Input: part model. Units: mm. Frame: model coordinates. A direction names the side the tool comes from. Coordinates: 2 decimals unless noted, no trailing zeros. Use one line per item in the form item = value.
from build123d import *

# Parameters (mm, degrees)
SKETCH_R              = 40
PAD_DEPTH             = 8
SKETCH001_R           = 1.5
POCKET_DEPTH          = 234.84015
POLARPATTERN_COUNT    = 12
SKETCH002_R           = 4
POCKET001_DEPTH       = 8.001
SKETCH003_R           = 8
POCKET002_DEPTH       = 1
SKETCH004_R           = 1.5
POCKET003_DEPTH       = 234.84015
POLARPATTERN001_COUNT = 6
FILLET_R              = 1
CHAMFER_SIZE          = 3.9
CHAMFER001_SIZE       = 3.9
CHAMFER002_SIZE       = 3.9
CHAMFER003_SIZE       = 3.9


with BuildPart() as part:
    # Sketch → Pad (new body)
    with BuildSketch(Plane.XY):
        Circle(SKETCH_R)
    extrude(amount=PAD_DEPTH)

    # Sketch001 → Pocket (cut, through all)
    with BuildSketch(Plane.XY.offset(8)):
        with Locations((34.5, 0)):
            Circle(SKETCH001_R)
    pocket = extrude(amount=-POCKET_DEPTH, mode=Mode.SUBTRACT)

    # PolarPattern: Pocket ×12 about axis
    polarpattern_axis = Axis((0, 0, 8), (0, 0, 1))
    for i in range(1, POLARPATTERN_COUNT):
        add(pocket.rotate(polarpattern_axis, i * 360 / POLARPATTERN_COUNT), mode=Mode.SUBTRACT)

    # Sketch002 → Pocket001 (cut, through all)
    with BuildSketch(Plane.XY.offset(8)):
        with Locations((11, 15)):
            Circle(SKETCH002_R)
        with Locations((11, -15)):
            Circle(SKETCH002_R)
        with Locations((-11, -15)):
            Circle(SKETCH002_R)
        with Locations((-11, 15)):
            Circle(SKETCH002_R)
    extrude(amount=-POCKET001_DEPTH, mode=Mode.SUBTRACT)

    # Sketch003 → Pocket002 (cut)
    with BuildSketch(Plane.XY.offset(8)):
        with Locations((11, 15)):
            Circle(SKETCH003_R)
        with Locations((-11, 15)):
            Circle(SKETCH003_R)
        with Locations((-11, -15)):
            Circle(SKETCH003_R)
        with Locations((11, -15)):
            Circle(SKETCH003_R)
    extrude(amount=-POCKET002_DEPTH, mode=Mode.SUBTRACT)

    # Sketch004 → Pocket003 (cut, through all)
    with BuildSketch(Plane.XY.offset(8)):
        with Locations((0, 24.738697)):
            Circle(SKETCH004_R)
    pocket003 = extrude(amount=-POCKET003_DEPTH, mode=Mode.SUBTRACT)

    # PolarPattern001: Pocket003 ×6 about axis
    polarpattern001_axis = Axis((0, 0, 8), (0, 0, 1))
    for i in range(1, POLARPATTERN001_COUNT):
        add(pocket003.rotate(polarpattern001_axis, i * 360 / POLARPATTERN001_COUNT), mode=Mode.SUBTRACT)

    # Fillet
    fillet_edges = [part.edges().sort_by_distance(p)[0] for p in [
        (-40, 0, 8),
    ]]
    fillet(fillet_edges, radius=FILLET_R)

    # Chamfer
    chamfer_edges = [part.edges().sort_by_distance(p)[0] for p in [
        (-15, 15, 7),
    ]]
    chamfer(chamfer_edges, length=CHAMFER_SIZE)

    # Chamfer001
    chamfer001_edges = [part.edges().sort_by_distance(p)[0] for p in [
        (7, 15, 7),
    ]]
    chamfer(chamfer001_edges, length=CHAMFER001_SIZE)

    # Chamfer002
    chamfer002_edges = [part.edges().sort_by_distance(p)[0] for p in [
        (-15, -15, 7),
    ]]
    chamfer(chamfer002_edges, length=CHAMFER002_SIZE)

    # Chamfer003
    chamfer003_edges = [part.edges().sort_by_distance(p)[0] for p in [
        (7, -15, 7),
    ]]
    chamfer(chamfer003_edges, length=CHAMFER003_SIZE)


solid = part.part
(1) Section query A-A on z = 1. State how many separate pieces and enclosed holes the cut face has, plus the area to 3 significant figures.
Computed:
separate_pieces = 1
enclosed_holes = 22
area = 4,700 mm^2
(2) Pull-direction query (X, two-part tool) for faces 3 (the cylindrical face through (-8.67, -39.05, 3.45)), 4 (the flat face through (-1, 1, 8)), 5 (the conical face through (-11.9, 10.9, 3.3)); classes: pulls with the +X half, pulls with the -X half, needs draft (parallel to the pull), parting line crosses it, or undercut.
Computed:
face_3 = parting line crosses it
face_4 = needs draft
face_5 = undercut
(3) First-contact query: pin 1 Ø9 at (x, y) = (11, 15) entering from -Z; pin 2 Ø1 at (y, z) = (1, 2.5) entering from -X; pin 3 Ø8 at (x, y) = (-10, 15.5) entering from +Z; pin 4 Ø3 at (x, z) = (-10.5, 2.5) entering from -Y. Flat tips, straight axial feed; report the tip coordinate or a pass-through.
Computed:
pin_1 = 0
pin_2 = -40
pin_3 = 4.22
pin_4 = -38.97
(4) Line query: probe 1 along Y at (x, z) = (-1, 5.5); probe 2 along Y at (x, z) = (-5, 6.75); probe 3 along Y at (x, z) = (22.5, 3). Output: solid intervals per line, ascending.
Computed:
probe_1 = -39.99 to -35.62, -33.38 to -25.86, -23.62 to 23.62, 25.86 to 33.38, 35.62 to 39.99
probe_2 = -39.69 to -19.75, -10.25 to 10.25, 19.75 to 39.69
probe_3 = -33.07 to -13.41, -11.32 to 11.32, 13.41 to 33.07
(5) Set-up query: faces 1 (the cylindrical face through (16.44, -31.14, 4.06)), 2 (the cylindrical face through (-3.37, -12.6, 7.51)). Return all of +Z, -Z, +X, -X, +Y, -Y with unobstructed straight access to the full face (end or side cutting, diameter ignored); none if empty.
Computed:
face_1 = +Z, -Z
face_2 = +Z
